Verification items for the finished model (mm, model axes). A direction names the side the tool comes from. Coordinates: 2 decimals unless noted, no trailing zeros. Loops run counter-clockwise (first coordinate to the right, second up) from the corner with the lowest first, then second, coordinate; pieces in that order, holes last.
Q1. Material ranges on probe 1 along X at (y, z) = (1, 8.5); probe 2 along X at (y, z) = (7.25, 6); probe 3 along X at (y, z) = (8.25, 6), recorded low to high.
Q2. Go/stop test with flat-tipped pins: P1, Ø3, axis at x = 4, z = 6.5, coming from the -Y side; P2, Ø2, axis at x = 26.22, z = 6, coming from the +Y side. Record where each tip stops, or that it passes through.
Q3. Mould release check, pull along X, two halves, no side actions. Record for faces 1 (the face through (2.305, 1.479, 3.39)), 2 (the face through (15, 3, 0)), 3 (the face through (24.7, 1.48, 8.59)), 4 (the face through (0, 5, 6)): +X half, -X half, draft (parallel to the pull), parting line (faces both ways), or undercut.
Q4. Sectioned sample at D-D (x = 4.25). Enter the section's corners in (y, z), then the cut area to 3 significant figures.
Q5. Sectioned sample at A-A (z = 6). Enter the section's corners in (x, y), then the cut area to 3 significant figures.
Q6. Sectioned sample at B-B (y = 5.5). Enter the section's corners in (x, z), then the cut area to 3 significant figures.
Q7. Sectioned sample at C-C (y = 2.5). Enter the section's corners in (x, z).
Q8. Access from +Z, -Z, +X, -X, +Y, -Y to the whole of each face (thin tool, end or side, straight path). Record for faces 5 (the face through (24.568, 6.549, 5.927)), 6 (the face through (0.784, 1, 6)).
Autodesk Inventor part; units mm, degrees
ref_plane "YZ Plane" through (0, 0, 0) normal (1, 0, 0) x (0, 1, 0)
ref_plane "XZ Plane" through (0, 0, 0) normal (0, 1, 0) x (-1, 0, 0)
ref_plane "XY Plane" through (0, 0, 0) normal (0, 0, 1) x (1, 0, 0)
sketch "Sketch1" plane through (0, 0, 0) normal (0, 0, 1) x (1, 0, 0)
  line L0 (0, 0) -> (30, 0)
  line L1 (30, 0) -> (30, 10)
  line L2 (30, 10) -> (0, 10) construction
  line L3 (0, 10) -> (0, 0)
  arc A0 (7.567, 10) -> (22.433, 10) centre (15, 11) ccw
  line L4 (0, 10) -> (7.567, 10)
  line L5 (22.433, 10) -> (30, 10)
  point P0 (15, 10)
  dimension "d0" = 30
  dimension "d1" = 10
  dimension "d2" = 15
  dimension "d3" = 1
extrude "Extrusion1" add sketch "Sketch1" along normal blind 12
sketch "Sketch2" plane through (0, 10, 0) normal (0, 1, 0) x (1, 0, 0)
  line L0 (0, 0) -> (0, -12) construction
  line L1 (7.567, -12) -> (0, -12) construction
  line L2 (30, -12) -> (22.433, -12) construction
  circle A0 centre (3.7835, -6) radius 1.65
  circle A1 centre (26.2165, -6) radius 1.65
  point P0 (0, -6)
  point P1 (3.7835, -12)
  point P2 (26.2165, -12)
  dimension "d6" = 3.3
  dimension "d7" = 3.3
extrude "Extrusion2" cut sketch "Sketch2" against normal blind 15
sketch "Sketch3" plane through (0, 0, 0) normal (0, -1, 0) x (1, 0, 0)
  circle A0 centre (3.7835, 6) radius 1.65 construction
  circle A1 centre (26.2165, 6) radius 1.65 construction
  line L0 (6.7835, 7.7321) -> (6.7835, 4.2679)
  line L1 (6.7835, 4.2679) -> (3.7835, 2.5359)
  line L2 (3.7835, 2.5359) -> (0.7835, 4.2679)
  line L3 (0.7835, 4.2679) -> (0.7835, 7.7321)
  line L4 (0.7835, 7.7321) -> (3.7835, 9.4641)
  line L5 (3.7835, 9.4641) -> (6.7835, 7.7321)
  line L6 (29.2165, 7.7321) -> (29.2165, 4.2679)
  line L7 (29.2165, 4.2679) -> (26.2165, 2.5359)
  line L8 (26.2165, 2.5359) -> (23.2165, 4.2679)
  line L9 (23.2165, 4.2679) -> (23.2165, 7.7321)
  line L10 (23.2165, 7.7321) -> (26.2165, 9.4641)
  line L11 (26.2165, 9.4641) -> (29.2165, 7.7321)
  point P0 (0, 0)
  dimension "d10" = 6
  dimension "d11" = 6
extrude "Extrusion3" cut sketch "Sketch3" against normal blind 3
equation "\"d6\" = d7"
properties part number "8mm Rod clamp"
Geometry check:
1. probe 1: x = 0 to 2.11, 5.45 to 24.55, 27.89 to 30
1. probe 2: x = 0 to 2.13, 5.43 to 8.5, 21.5 to 24.57, 27.87 to 30
1. probe 3: x = 0 to 2.13, 5.43 to 8.02, 21.98 to 24.57, 27.87 to 30
2. P1: stops at y = 3
2. P2: passes through
3. face 1: undercut
3. face 2: draft
3. face 3: undercut
3. face 4: -X half
4. outline: (0, 0) - (10, 0) - (10, 4.42) - (3, 4.42) - (3, 2.81) - (0, 2.81) - close; (0, 9.19) - (3, 9.19) - (3, 7.58) - (10, 7.58) - (10, 12) - (0, 12) - close
4. area: 78.7 mm2
5. outline: (0, 0) - (0.78, 0) - (0.78, 3) - (2.13, 3) - (2.13, 10) - (0, 10) - close; (5.43, 3) - (6.78, 3) - (6.78, 0) - (23.22, 0) - (23.22, 3) - (24.57, 3) - (24.57, 10) - (22.43, 10) arc R7.5 cw to (7.57, 10) - (5.43, 10) - close; (27.87, 3) - (29.22, 3) - (29.22, 0) - (30, 0) - (30, 10) - (27.87, 10) - close
5. area: 144 mm2
6. outline: (0, 0) - (9.9, 0) - (9.9, 12) - (0, 12) - close; (20.1, 0) - (30, 0) - (30, 12) - (20.1, 12) - close; hole circle Ø3.3 at (3.78, 6); hole circle Ø3.3 at (26.22, 6)
6. area: 221 mm2
7. outline: (0, 0) - (30, 0) - (30, 12) - (0, 12) - close; hole (0.78, 4.27) - (3.78, 2.54) - (6.78, 4.27) - (6.78, 7.73) - (3.78, 9.46) - (0.78, 7.73) - close; hole (23.22, 4.27) - (26.22, 2.54) - (29.22, 4.27) - (29.22, 7.73) - (26.22, 9.46) - (23.22, 7.73) - close
8. face 5: +Y, -Y
8. face 6: -Y
